For this review, take the finished solid that the model builds, in its own axes (mm). A direction names the side the tool comes from. Coordinates: 2 decimals unless noted, no trailing zeros. Loops run counter-clockwise (first coordinate to the right, second up) from the corner with the lowest first, then second, coordinate; pieces in that order, holes last. Notation, with made-up numbers: (31, 64.5) - (43, 64.5) arc R6 ccw to (43, 74.5) - close; hole circle Ø4 at (-33.5, -9.75). An arc over 180 degrees is marked (long way). Use one line per item in the form item = value. Start each with the question number.
1. Add section A-A on y = 28. Count the separate pieces of the cut face and the enclosed holes in it, and give its area (3 significant figures).
2. Machinability: for faces 1 (the face through (25.75, 34, -145)), 2 (the face through (-1, 33, -47.5)), 3 (the face through (18.495, 8.676, 126.996)), which of the approach directions +Z, -Z, +X, -X, +Y, -Y give a long, thin tool a straight path to every point of the face, cutting with its end or side? Answer none if there is none.
3. To check wall thickness, follow probe 1 along Y at (x, z) = (19, -177); probe 2 along Z at (x, y) = (28, 58); probe 3 along Z at (x, y) = (22, 15.5). State the ranges of each line that lie inside material, in increasing order.
4. For pin 1 Ø1 at (x, y) = (-24.5, 49.5) entering from -Z; pin 2 Ø2.5 at (x, y) = (-16.5, 18.5) entering from +Z; pin 3 Ø3.5 at (y, z) = (18, -85.5) entering from -X; pin 4 Ø1.5 at (x, y) = (-17.5, 4.5) entering from -Z, all flat-tipped, find the tip position at first contact; note any pin that passes through.
5. Add section C-C on x = -4.5. Give the boundary of the cut face in (y, z), and give its area (3 significant figures).
6. Add section B-B on z = -145. Give the boundary of the cut face in (x, y), and give its area (4 significant figures).
7. Add section D-D on z = 131. Give the boundary of the cut face in (x, y), and give its area (4 significant figures).
8. Draft analysis for pull direction X (two halves, no side actions). For faces 4 (the face through (-17.899, 33.031, 31.783)), 5 (the face through (25.75, 34, 5)), 6 (the face through (3.755, 33.031, 11.923)), 7 (the face through (33, 26, -60)), state which applies: +X half, -X half, draft (parallel to the pull), parting line (faces both ways), or undercut.
```python
from build123d import *

# Parameters (mm, degrees)
SKETCH1_R           = 12.5
SKETCH1_R_2         = 3
BOSS_EXTRUDE1_DEPTH = 67
SKETCH2_R           = 4
CUT_EXTRUDE1_DEPTH  = 212.501773042
FILLET1_R           = 15
CUT_EXTRUDE3_REACH  = 218.502
CUT_EXTRUDE3_START  = -5
SKETCH3_W           = 45
SKETCH3_H           = 45
SKETCH3_R           = 2
SKETCH3_R_2         = 12.5
SKETCH3_2_R         = 2
SKETCH3_2_R_2       = 12.5
CUT_EXTRUDE4_DEPTH  = 212.501773075
SKETCH3_4_R         = 12.5
CUT_EXTRUDE5_DEPTH  = 10


with BuildPart() as part:
    # Sketch1 → Boss-Extrude1 (new body)
    with BuildSketch(Plane(origin=(0, 0, 0), x_dir=(1, 0, 0), z_dir=(0, 1, 0))):
        Polygon((0.75, -188), (35.75, -188), (35.75, 188), (0.75, 188), (0.75, 75), (-34.25, 75), (-34.25, -75), (0.75, -75), align=None)
        with Locations(Location((0, 0, 0), (0, 0, 270))):
            Circle(SKETCH1_R, mode=Mode.SUBTRACT)
        with Locations(Location((-16.75, -29.011851027, 0), (0, 0, 270))):
            Circle(SKETCH1_R_2, mode=Mode.SUBTRACT)
        with Locations(Location((16.75, -29.011851027, 0), (0, 0, 270))):
            Circle(SKETCH1_R_2, mode=Mode.SUBTRACT)
        with Locations(Location((16.75, 29.011851027, 0), (0, 0, 270))):
            Circle(SKETCH1_R_2, mode=Mode.SUBTRACT)
        with Locations(Location((-16.75, 29.011851027, 0), (0, 0, 270))):
            Circle(SKETCH1_R_2, mode=Mode.SUBTRACT)
    extrude(amount=BOSS_EXTRUDE1_DEPTH)

    # Sketch2 → Cut-Extrude1 (cut, through all)
    with BuildSketch(Plane(origin=(35.75, 0, 0), x_dir=(0, 0, -1), z_dir=(1, 0, 0))):
        with Locations((-177, 58.5)):
            Circle(SKETCH2_R)
        with Locations((-123, 58.5)):
            Circle(SKETCH2_R)
        with Locations((-177, 8.5)):
            Circle(SKETCH2_R)
        with Locations((-123, 8.5)):
            Circle(SKETCH2_R)
        with Locations((177, 58.5)):
            Circle(SKETCH2_R)
        with Locations((177, 8.5)):
            Circle(SKETCH2_R)
        with Locations((123, 8.5)):
            Circle(SKETCH2_R)
        with Locations((123, 58.5)):
            Circle(SKETCH2_R)
    extrude(amount=-CUT_EXTRUDE1_DEPTH, mode=Mode.SUBTRACT)

    # Fillet1
    fillet1_edges = [part.edges().sort_by_distance(p)[0] for p in [
        (0.75, 33.5, 75),
        (-34.25, 33.5, 75),
        (-34.25, 33.5, -75),
        (0.75, 33.5, -75),
    ]]
    fillet(fillet1_edges, radius=FILLET1_R)

    # Cut-Extrude3: up to this face of the body (flat: up to its plane)
    cut_extrude3_end = Plane(part.part.faces().sort_by_distance((-34.25, 33.5, 0))[0])
    # Sketch3 → Cut-Extrude3 (cut, up to the picked face)
    with BuildSketch(Plane(origin=(35.75, 0, 0), x_dir=(0, 0, -1), z_dir=(1, 0, 0)).offset(CUT_EXTRUDE3_START), mode=Mode.PRIVATE) as cut_extrude3_sk1:
        with Locations((70, 33.5)):
            Rectangle(SKETCH3_W, SKETCH3_H)
        with Locations((54.5, 49)):
            Circle(SKETCH3_R, mode=Mode.SUBTRACT)
        with Locations((54.5, 18)):
            Circle(SKETCH3_R, mode=Mode.SUBTRACT)
        with Locations((85.5, 18)):
            Circle(SKETCH3_R, mode=Mode.SUBTRACT)
        with Locations((85.5, 49)):
            Circle(SKETCH3_R, mode=Mode.SUBTRACT)
        with Locations((70, 33.5)):
            Circle(SKETCH3_R_2, mode=Mode.SUBTRACT)
    cut_extrude3_tool1 = split(extrude(cut_extrude3_sk1.sketch, amount=-CUT_EXTRUDE3_REACH, mode=Mode.PRIVATE), bisect_by=cut_extrude3_end, keep=Keep.BOTH, mode=Mode.PRIVATE)
    add(cut_extrude3_tool1.solids().sort_by(Axis((30.75, 11.636396, -70), (-1, 0, 0)))[0], mode=Mode.SUBTRACT)

    # Sketch3<2> → Cut-Extrude4 (cut, through all)
    with BuildSketch(Plane(origin=(35.75, 0, 0), x_dir=(0, 0, -1), z_dir=(1, 0, 0))):
        with Locations((54.5, 49)):
            Circle(SKETCH3_2_R)
        with Locations((85.5, 49)):
            Circle(SKETCH3_2_R)
        with Locations((85.5, 18)):
            Circle(SKETCH3_2_R)
        with Locations((54.5, 18)):
            Circle(SKETCH3_2_R)
        with Locations((70, 33.5)):
            Circle(SKETCH3_2_R_2)
    extrude(amount=-CUT_EXTRUDE4_DEPTH, mode=Mode.SUBTRACT)

    # Sketch3<4> → Cut-Extrude5 (cut)
    with BuildSketch(Plane(origin=(35.75, 0, 0), x_dir=(0, 0, -1), z_dir=(1, 0, 0))):
        with Locations((-5, 33.5)):
            Circle(SKETCH3_4_R)
        with Locations((145, 33.5)):
            Circle(SKETCH3_4_R)
    extrude(amount=-CUT_EXTRUDE5_DEPTH, mode=Mode.SUBTRACT)


solid = part.part
```
Conclusion:
q1.separate_pieces = 2
q1.enclosed_holes = 5
q1.area = 14,900 mm^2
q2.face_1 = +X
q2.face_2 = -X
q2.face_3 = +X, -X
q3.probe_1 = 0 to 4.5, 12.5 to 54.5, 62.5 to 67
q3.probe_2 = -188 to -180.97, -173.03 to -126.97, -119.03 to 119.03, 126.97 to 173.03, 180.97 to 188
q3.probe_3 = -188 to -92.5, -47.5 to 188
q4.pin_1 = -47.5
q4.pin_2 = 75
q4.pin_3 = through
q4.pin_4 = -75
q5.outline = (0, -78.6) - (11, -78.6) - (11, -47.5) - (56, -47.5) - (56, -78.6) - (67, -78.6) - (67, -11.66) - (0, -11.66) - close; (0, 11.66) - (67, 11.66) - (67, 78.6) - (0, 78.6) - close
q5.area = 7,570 mm^2
q6.outline = (0.75, 0) - (35.75, 0) - (35.75, 21) - (25.75, 21) - (25.75, 46) - (35.75, 46) - (35.75, 67) - (0.75, 67) - close
q6.area = 2,095 mm^2
q7.outline = (0.75, 0) - (35.75, 0) - (35.75, 67) - (0.75, 67) - close
q7.area = 2,345 mm^2
q8.face_4 = undercut
q8.face_5 = +X half
q8.face_6 = undercut
q8.face_7 = draft
